Source: CAD feature listing. Evaluate the final solid. Frame: model axes, mm. Face numbers are marked on the shaded views. A direction names the side the tool comes from. Give positions to 0.01 mm unless a question says otherwise; leave off trailing zeros. Loops run counter-clockwise (first coordinate to the right, second up) from the corner with the lowest first, then second, coordinate; pieces in that order, holes last. Notation, with made-up numbers: (69.5, 76) - (93.5, 76) arc R28 ccw to (93.5, 95) - close; hole circle Ø2 at (45.5, 8). An arc over 180 degrees is marked (long way). Put each result on its own line as item: value.
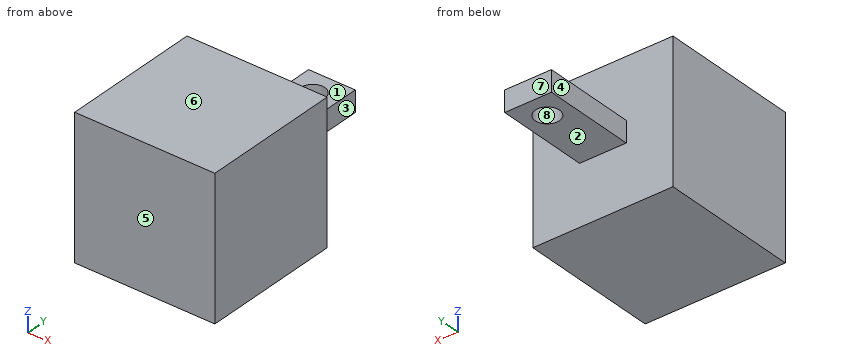
Autodesk Inventor part; units mm, degrees
ref_plane "YZ Plane" through (0, 0, 0) normal (1, 0, 0) x (0, 1, 0)
ref_plane "XZ Plane" through (0, 0, 0) normal (0, 1, 0) x (-1, 0, 0)
ref_plane "XY Plane" through (0, 0, 0) normal (0, 0, 1) x (1, 0, 0)
sketch "Sketch1" plane through (0, 0, 0) normal (0, 1, 0) x (-1, 0, 0)
  line L0 (0, 0) -> (30, 0)
  line L1 (30, 0) -> (30, -30)
  line L2 (30, -30) -> (0, -30)
  line L3 (0, -30) -> (0, 0)
  dimension "d0" = 30
  dimension "d1" = 30
extrude "Extrusion1" add sketch "Sketch1" along normal blind 30
sketch "Sketch2" plane through (0, 30, 0) normal (0, 1, 0) x (1, 0, 0)
  line L0 (-20, 17.25) -> (-10, 17.25)
  line L1 (-10, 17.25) -> (-10, 12.75)
  line L2 (-10, 12.75) -> (-20, 12.75)
  line L3 (-20, 12.75) -> (-20, 17.25)
  line L4 (-20, 17.25) -> (-10, 12.75) construction
  line L5 (-10, 17.25) -> (-20, 12.75) construction
  line L6 (-30, 30) -> (-30, 0)
  line L7 (-30, 0) -> (0, 0)
  point P0 (-15, 15)
  point P1 (-30, 15)
  dimension "d4" = 15
  dimension "d5" = 15
  dimension "d6" = 10
  dimension "d7" = 4.5
extrude "Extrusion2" add sketch "Sketch2" along normal blind 20
sketch "Sketch3" plane through (-20, 30, -12.75) normal (0, 0, 1) x (1, 0, 0)
  circle A0 centre (5, 14.8617) radius 2.6
  point P0 (20, -30)
  dimension "d10" = 5.2
extrude "Extrusion3" cut sketch "Sketch3" against normal blind 20
properties part number "ObjectCube"
1) Section query A-A, the plane x = -15. Output: boundary loops of the cut face in (y, z), plus the area to 3 significant figures.
Check result:
outline: (0, -30) - (30, -30) - (30, -17.25) - (42.26, -17.25) - (42.26, -12.75) - (30, -12.75) - (30, 0) - (0, 0) - close; (47.46, -17.25) - (50, -17.25) - (50, -12.75) - (47.46, -12.75) - close
area: 967 mm²
2) Access query for the marked faces 1, 2, 3 and 4. Directions: +Z, -Z, +X, -X, +Y, -Y. A direction counts if a zero-diameter tool reaches every point of the face in a straight line with its end or side. Return the directions, or none.
Check result:
face 1: +Z, +X, -X, +Y
face 2: -Z, +X, -X, +Y
face 3: +Z, -Z, +X, +Y
face 4: +Z, -Z, -X, +Y
3) Section query C-C, the plane z = -15.5. Output: boundary loops of the cut face in (x, y), plus the area to 3 significant figures.
Check result:
outline: (-30, 0) - (0, 0) - (0, 30) - (-10, 30) - (-10, 50) - (-20, 50) - (-20, 30) - (-30, 30) - close; hole circle Ø5.2 at (-15, 44.86)
area: 1,080 mm²
4) Pin query (flat end, axial travel): P1, Ø1.3, axis at y = 45, z = -14, coming from the -X side; P2, Ø3, axis at x = -15.5, y = 37.5, coming from the -Z side; P3, Ø8.5, axis at x = -15, y = 44.86, coming from the +Z side. Return the tip coordinate at first contact, or that it passes through.
Check result:
P1: x = -20
P2: z = -17.25
P3: z = -12.75
5) Mould query, pull axis Y, two halves, no side actions, for the marked faces 5, 6, 7 and 8. Classes: pulls with the +Y half, pulls with the -Y half, needs draft (parallel to the pull), parting line crosses it, or undercut.
Check result:
face 5: pulls with the -Y half
face 6: needs draft
face 7: pulls with the +Y half
face 8: undercut
6) Section query D-D, the plane z = -19.5. Output: boundary loops of the cut face in (x, y).
Check result:
outline: (-30, 0) - (0, 0) - (0, 30) - (-30, 30) - close
7) Material intervals for line 1 along Y through (x, z) = (-15, -14.65); line 2 along Y through (x, z) = (-6.5, -20.5); line 3 along Z through (x, y) = (-18.5, 46.5), sorted ascending. Write a range as [from, to].
Check result:
line 1: [0, 42.26], [47.46, 50]
line 2: [0, 30]
line 3: [-17.25, -12.75]
8) Section query B-B, the plane y = 44. Output: boundary loops of the cut face in (x, z), plus the area to 3 significant figures.
Check result:
outline: (-20, -17.25) - (-17.45, -17.25) - (-17.45, -12.75) - (-20, -12.75) - close; (-12.55, -17.25) - (-10, -17.25) - (-10, -12.75) - (-12.55, -12.75) - close
area: 22.9 mm²
